```python
from build123d import *

# Parameters (mm, degrees)
SKETCH_W            = 533.4
SKETCH_H            = 279.4
EXTRUDE_2_DEPTH     = 6.35
EXTRUDE4_DEPTH      = 0.508
EXTRUDE4_DEPTH_BACK = 0.508
EXTRUDE5_DEPTH      = 76.2
EXTRUDE6_DEPTH      = 6.35
CUT_EXTRUDE1_DEPTH  = 23.368


with BuildPart() as part:
    # Sketch → Extrude 2 (new body)
    with BuildSketch(Plane(origin=(0, 0, 0), x_dir=(1, 0, 0), z_dir=(0, 1, 0))):
        with Locations((266.7, 139.7)):
            Rectangle(SKETCH_W, SKETCH_H)
    extrude(amount=EXTRUDE_2_DEPTH)

    # Sketch5 → Extrude4 (add, two sides: drawn at the far end of the back side and taken through both)
    with BuildSketch(Plane.ZY.offset(-266.7).offset(-EXTRUDE4_DEPTH_BACK)):
        with BuildLine():
            Line((0, 6.35), (10.16, 6.35))
            ThreePointArc((10.16, 6.35), (17.145, 13.335), (10.16, 20.32))
            Line((10.16, 20.32), (10.16, 19.685))
            ThreePointArc((10.16, 19.685), (16.509592253, 13.406959845), (10.303910448, 6.986630935))
            Line((10.303910448, 6.986630935), (-17.78, 6.35))
            Line((-17.78, 6.35), (0, 6.35))
        make_face()
    extrude(amount=EXTRUDE4_DEPTH + EXTRUDE4_DEPTH_BACK)

    # Sketch6 → Extrude5 (cut)
    with BuildSketch(Plane.XZ):
        Polygon((185.553034717, -266.27947971), (177.8, -279.4), (185.42, -279.4), (533.4, -279.4), (533.4, 0), (342.9, 0), align=None)
        Polygon((0, 0), (203.2, 0), (0, -279.4), align=None)
    extrude(amount=-EXTRUDE5_DEPTH, mode=Mode.SUBTRACT)

    # Sketch7 → Extrude6 (add)
    with BuildSketch(Plane(origin=(254.155589587, 0, -150.182848392), x_dir=(-0.5087293121266415, 0, -0.8609265282143153), z_dir=(0.8609265282143153, 0, -0.5087293121266415))):
        Polygon((-161.743281128, 6.35), (-62.577151256, 85.691531912), (67.540800287, 6.35), align=None)
    extrude(amount=-EXTRUDE6_DEPTH)

    # Sketch8 → Cut-Extrude1 (cut)
    with BuildSketch(Plane(origin=(254.155589587, 0, -150.182848392), x_dir=(-0.5087293121266415, 0, -0.8609265282143153), z_dir=(0.8609265282143153, 0, -0.5087293121266415))):
        Polygon((-96.293635413, 58.715411062), (-30.684203238, 66.244289445), (-62.577151256, 85.691531912), align=None)
    extrude(amount=-CUT_EXTRUDE1_DEPTH, mode=Mode.SUBTRACT)


solid = part.part
```
Work out the finished part from the listing and answer in its coordinate system (mm). A direction names the side the tool comes from. Coordinates: 2 decimals unless noted, no trailing zeros. Order: outer loops, then holes, each group sorted by start corner. A loop starts at its lowest first (then second) coordinate and runs counter-clockwise, first axis right, second up. Notation, with made-up numbers: (4, 72) - (55, 72) arc R32 ccw to (55, 99) - close; hole circle Ø9 at (5.25, -21). An arc over 180 degrees is marked (long way). Answer as a JSON object with one key per item and string values.
1. Consider line 1 (Y direction, x = 210.5, z = -196); line 2 (X direction, y = 24, z = -153.5); line 3 (Z direction, x = 253.5, y = 50.5). Determine where each line is inside the solid, lowest interval first.
Output values:
{"line 1": "y = 0 to 6.35", "line 2": "x = 244.82 to 252.2", "line 3": "z = -144.15 to -138.81"}
2. A tool of negligible diameter and unlimited length cuts with its end or side. For faces 4 (the face through (266.192, 6.6, 9.9)), 5 (the face through (266.707, 13.181, 17.143)), from which of +Z, -Z, +X, -X, +Y, -Y can it reach the whole face along a straight path? Write none if from no direction.
Output values:
{"face 4": "+Z, -X, +Y", "face 5": "+Z, +X, -X"}
3. The mould has two halves that part along Z. Classify faces 1 (the face through (169, 0, -142)), 2 (the face through (283.993, 62.427, -93.536)), 3 (the face through (242.44, 36.72, -163.86)): +Z half, -Z half, draft (parallel to the pull), parting line (faces both ways), or undercut.
Output values:
{"face 1": "draft", "face 2": "+Z half", "face 3": "-Z half"}
4. Find section D-D on z = -142.5. Determine the outline of the cut face in (x, y), plus the area to 3 significant figures.
Output values:
{"outline": "(99.56, 0) - (258.7, 0) - (258.7, 52.98) - (251.32, 50.69) - (251.32, 6.35) - (99.56, 6.35) - close", "area": "1,350 mm²"}
5. Each of these flat-tipped pins is pushed along its axis until it touches: P1, Ø1.1, axis at x = 266.5, z = 4, coming from the -Y side; P2, Ø0.7, axis at x = 266.5, y = 20, coming from the -Z side; P3, Ø10, axis at x = 255, z = -87, coming from the -Y side; P4, Ø5, axis at x = 244, y = 3.5, coming from the +Z side. Where does it stop, or does it pass through?
Output values:
{"P1": "stops at y = 6.35", "P2": "stops at z = -129.88", "P3": "stops at y = 0", "P4": "stops at z = 0"}
6. Find section C-C on y = 51. Determine the outline of the cut face in (x, z), plus the area to 3 significant figures.
Output values:
{"outline": "(251.58, -142.06) - (257.05, -145.29) - (308.05, -58.98) - (302.58, -55.75) - close", "area": "637 mm²"}
7. Find section A-A on z = -74. Determine the outline of the cut face in (x, y).
Output values:
{"outline": "(149.38, 0) - (299.17, 0) - (299.17, 59.61) - (291.8, 60.04) - (291.8, 6.35) - (149.38, 6.35) - close"}
8. Find section B-B on x = 173.5. Determine the outline of the cut face in (y, z), plus the area to 3 significant figures.
Output values:
{"outline": "(0, -279.4) - (6.35, -279.4) - (6.35, -40.84) - (0, -40.84) - close", "area": "1,510 mm²"}
